CAD build for the part. Positions are in the model's coordinates, mm. Coordinates: 2 decimals unless noted, no trailing zeros. Write each loop counter-clockwise with the first axis right and the second up, starting at its lowest first coordinate (ties: lowest second). Pieces come first, ordered by that corner, then holes. Notation, with made-up numbers: M 28,59.25 L 43,59.25 A23 ccw 43,88.25 Z; hole C 53.5,66 d1. An arc over 180 degrees is marked long. Answer as CSV lines item,"result". Start each with the question number.
```python
from build123d import *

# Parameters (mm, degrees)
BOSS_EXTRUDE2_DEPTH                                  = 8
CSK_FOR_M3_HEX_SOCKET_COUNTERSUNK_CAP_SC_D           = 3.4
CSK_FOR_M3_HEX_SOCKET_COUNTERSUNK_CAP_SC_CSINK_D     = 6.72
CSK_FOR_M3_HEX_SOCKET_COUNTERSUNK_CAP_SC_CSINK_ANGLE = 90


with BuildPart() as part:
    # Sketch3 → Boss-Extrude2 (new body)
    with BuildSketch(Plane(origin=(0, 0, 0), x_dir=(1, 0, 0), z_dir=(0, 1, 0))):
        with BuildLine():
            Line((-50, 40), (50, 40))
            ThreePointArc((50, 40), (57.071067812, 37.071067812), (60, 30))
            Line((60, 30), (60, -30))
            ThreePointArc((60, -30), (57.071067812, -37.071067812), (50, -40))
            Line((50, -40), (-50, -40))
            ThreePointArc((-50, -40), (-57.071067812, -37.071067812), (-60, -30))
            Line((-60, -30), (-60, 30))
            ThreePointArc((-60, 30), (-57.071067812, 37.071067812), (-50, 40))
        make_face()
    extrude(amount=BOSS_EXTRUDE2_DEPTH)

    # CSK for M3 Hex Socket Countersunk Cap Screw1 (through all)
    with Locations(Plane(origin=(0, 8, 0), x_dir=(1, 0, 0), z_dir=(0, 1, 0))):
        with Locations((0, 0), (0, 10), (0, 25), (20, 10), (20, 0), (45, 0), (45, 25), (-45, 25), (-45, 0), (-20, 10), (-20, 0), (-20, -10), (-45, -25), (45, -25), (20, -10), (0, -25), (0, -10)):
            CounterSinkHole(CSK_FOR_M3_HEX_SOCKET_COUNTERSUNK_CAP_SC_D / 2, CSK_FOR_M3_HEX_SOCKET_COUNTERSUNK_CAP_SC_CSINK_D / 2, counter_sink_angle=CSK_FOR_M3_HEX_SOCKET_COUNTERSUNK_CAP_SC_CSINK_ANGLE)


solid = part.part
```
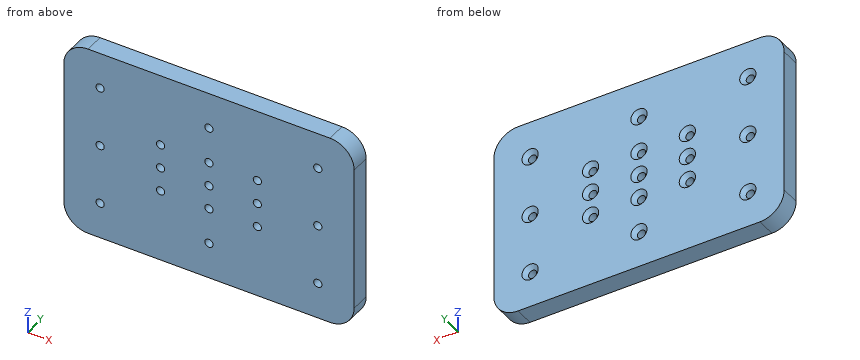
1) Band-saw the part on B-B, the plane x = -45. List the corners of the cut face in (y, z), plus the area to 3 significant figures.
2) Pin check, flat tip, straight feed: P1, Ø4, axis at x = 45, z = -25, coming from the +Y side. Stop position of the tip, or through.
3) Band-saw the part on C-C, the plane z = 25. List the corners of the cut face in (x, y).
4) Band-saw the part on A-A, the plane y = 3. State how many separate pieces and enclosed holes the cut face has, plus the area to 3 significant figures.
5) Probe L1, parallel to Z at x = -20, y = 2.25; L2, parallel to Z at x = -45, y = 2.75; L3, parallel to X at y = 3.5, z = -25. List the from-to ranges inside material, lowest first. Write a range as [from, to].
Result sheet:
1,outline,"M 0,-40 L 8,-40 L 8,-28.36 L 6.34,-26.7 L 0,-26.7 Z; M 0,-23.3 L 6.34,-23.3 L 8,-21.64 L 8,-3.36 L 6.34,-1.7 L 0,-1.7 Z; M 0,1.7 L 6.34,1.7 L 8,3.36 L 8,21.64 L 6.34,23.3 L 0,23.3 Z; M 0,26.7 L 6.34,26.7 L 8,28.36 L 8,40 L 0,40 Z"
1,area,"550 mm²"
2,P1,"stops at y = 6.64"
3,outline,"M -60,0 L -46.7,0 L -46.7,6.34 L -48.36,8 L -60,8 Z; M -43.3,0 L -1.7,0 L -1.7,6.34 L -3.36,8 L -41.64,8 L -43.3,6.34 Z; M 1.7,0 L 43.3,0 L 43.3,6.34 L 41.64,8 L 3.36,8 L 1.7,6.34 Z; M 46.7,0 L 60,0 L 60,8 L 48.36,8 L 46.7,6.34 Z"
4,separate pieces,"1"
4,enclosed holes,"17"
4,area,"9,360 mm²"
5,L1,"z = [-40, -11.7], [-8.3, -1.7], [1.7, 8.3], [11.7, 40]"
5,L2,"z = [-40, -26.7], [-23.3, -1.7], [1.7, 23.3], [26.7, 40]"
5,L3,"x = [-60, -46.7], [-43.3, -1.7], [1.7, 43.3], [46.7, 60]"
